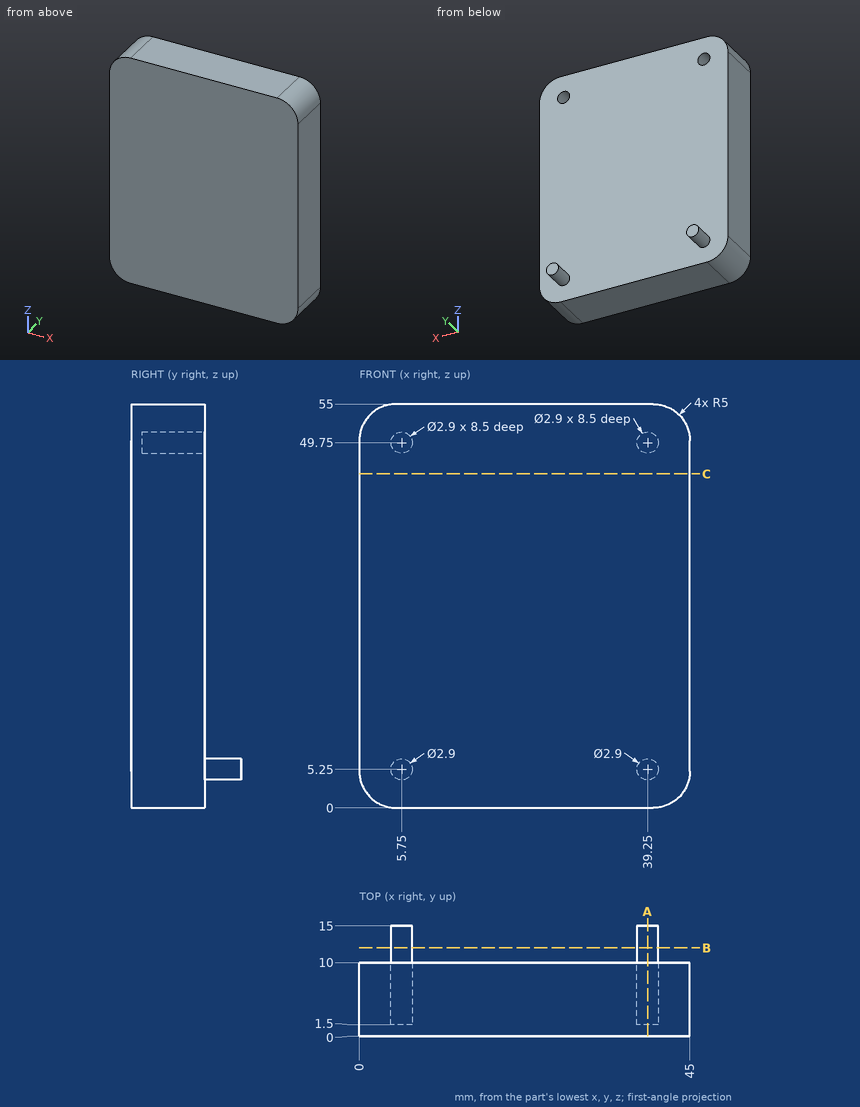
Design review of the part shown in the three views and the two pictorial views. Dimensions are in mm from the part's minimum x, y and z. Round coordinates to 2 decimals unless told otherwise and drop trailing zeros. Write each loop counter-clockwise with the first axis right and the second up, starting at its lowest first coordinate (ties: lowest second). Pieces come first, ordered by that corner, then holes. Notation, with made-up numbers: (73.25, -1) - (98.25, -1) arc R25 cw to (98.25, 33) - close; hole circle Ø4 at (-9, 74.5). An arc over 180 degrees is marked (long way). Return JSON: item names as keys, results as strings. Group by question number.
Item 1: We need section A-A on x = 39.25. Write out the cut boundary in (y, z).
Item 2: We need section C-C on z = 45.5. Write out the cut boundary in (x, y), and give its area (3 significant figures).
Item 3: We need section B-B on y = 12. Write out the cut boundary in (x, z), and give its area (3 significant figures).
Item 4: Insertion check: P1, Ø2.5, axis at x = 39, z = 50, coming from the +Y side; P2, Ø6, axis at x = 23.5, y = 9.5, coming from the -Z side; P3, Ø2.5, axis at x = 39.25, z = 49.75, coming from the +Y side. Each pin has a flat end and moves straight along its axis. Give the tip position at first contact, or say it passes through.
Item 5: For probe 1 along X at (y, z) = (4, 49.75); probe 2 along Z at (x, y) = (5.75, 4.75); probe 3 along Y at (x, z) = (34, 13), list the stretches that pass through material, from the lowest coordinate up. Write a range as [from, to].
Model answer:
{
 "1": {"outline": "(0, 0) - (10, 0) - (10, 3.8) - (15, 3.8) - (15, 6.7) - (10, 6.7) - (10, 48.3) - (1.5, 48.3) - (1.5, 51.2) - (10, 51.2) - (10, 55) - (0, 55) - close"},
 "2": {"outline": "(0, 0) - (45, 0) - (45, 10) - (0, 10) - close", "area": "450 mm²"},
 "3": {"outline": "circle Ø2.9 at (5.75, 5.25); circle Ø2.9 at (39.25, 5.25)", "area": "13.2 mm²"},
 "4": {"P1": "stops at y = 10", "P2": "stops at z = 0", "P3": "stops at y = 1.5"},
 "5": {"probe 1": "x = [0, 4.3], [7.2, 37.8], [40.7, 45]", "probe 2": "z = [0, 48.3], [51.2, 55]", "probe 3": "y = [0, 10]"}
}
